from build123d import *

# Parameters (mm, degrees)
SKETCH1_W           = 95
SKETCH1_H           = 83
BOSS_EXTRUDE1_DEPTH = 3
SKETCH3_W           = 95
SKETCH3_H           = 83
SKETCH3_W_2         = 89
SKETCH3_H_2         = 77
BOSS_EXTRUDE2_DEPTH = 9.5
SKETCH4_W           = 6
SKETCH4_H           = 6
BOSS_EXTRUDE3_DEPTH = 9.5
FILLET1_R           = 5
SKETCH5_R           = 1.5
CUT_EXTRUDE1_DEPTH  = 12.5
BOSS_EXTRUDE4_DEPTH = 3
SKETCH7_W           = 12.5
SKETCH7_H           = 3
SKETCH7_W_2         = 10
CUT_EXTRUDE2_DEPTH  = 1.3
SKETCH8_W           = 86
SKETCH8_H           = 5.5
SKETCH8_W_2         = 48.5
SKETCH8_H_2         = 4
SKETCH8_W_3         = 39.36
CUT_EXTRUDE3_DEPTH  = 3
SKETCH10_W          = 10.8
SKETCH10_H          = 3
SKETCH10_W_2        = 13.5
CUT_EXTRUDE4_DEPTH  = 3
SKETCH11_R          = 1.5
CUT_EXTRUDE5_DEPTH  = 3


with BuildPart() as part:
    # Sketch1 → Boss-Extrude1 (new body)
    with BuildSketch(Plane(origin=(0, 0, 0), x_dir=(1, 0, 0), z_dir=(0, 1, 0))):
        with Locations((47.5, 41.5)):
            Rectangle(SKETCH1_W, SKETCH1_H)
    extrude(amount=BOSS_EXTRUDE1_DEPTH)

    # Sketch3 → Boss-Extrude2 (add)
    with BuildSketch(Plane(origin=(0, 3, 0), x_dir=(1, 0, 0), z_dir=(0, 1, 0))):
        with Locations((47.5, 41.5)):
            Rectangle(SKETCH3_W, SKETCH3_H)
        with Locations((47.5, 41.5)):
            Rectangle(SKETCH3_W_2, SKETCH3_H_2, mode=Mode.SUBTRACT)
    extrude(amount=BOSS_EXTRUDE2_DEPTH)

    # Sketch4 → Boss-Extrude3 (add)
    with BuildSketch(Plane(origin=(0, 3, 0), x_dir=(1, 0, 0), z_dir=(0, 1, 0))):
        with Locations((6, 77)):
            Rectangle(SKETCH4_W, SKETCH4_H)
        with Locations((6, 6)):
            Rectangle(SKETCH4_W, SKETCH4_H)
        with Locations((89, 6)):
            Rectangle(SKETCH4_W, SKETCH4_H)
        with Locations((89, 77)):
            Rectangle(SKETCH4_W, SKETCH4_H)
    extrude(amount=BOSS_EXTRUDE3_DEPTH)

    # Fillet1
    fillet1_edges = [part.edges().sort_by_distance(p)[0] for p in [
        (0, 6.25, -83),
        (95, 6.25, -83),
        (95, 6.25, 0),
        (0, 6.25, 0),
    ]]
    fillet(fillet1_edges, radius=FILLET1_R)

    # Sketch5 → Cut-Extrude1 (cut)
    with BuildSketch(Plane(origin=(0, 12.5, 0), x_dir=(1, 0, 0), z_dir=(0, 1, 0))):
        with Locations(Location((5, 78, 0), (0, 0, 270))):
            Circle(SKETCH5_R)
        with Locations(Location((90, 78, 0), (0, 0, 270))):
            Circle(SKETCH5_R)
        with Locations(Location((90, 5, 0), (0, 0, 270))):
            Circle(SKETCH5_R)
        with Locations(Location((5, 5, 0), (0, 0, 270))):
            Circle(SKETCH5_R)
    extrude(amount=-CUT_EXTRUDE1_DEPTH, mode=Mode.SUBTRACT)

    # Sketch6 → Boss-Extrude4 (add)
    with BuildSketch(Plane(origin=(0, 12.5, 0), x_dir=(1, 0, 0), z_dir=(0, 1, 0))):
        with BuildLine():
            Line((5, 0), (90, 0))
            ThreePointArc((90, 0), (93.535533906, 1.464466094), (95, 5))
            Line((95, 5), (95, 78))
            ThreePointArc((95, 78), (93.535533906, 81.535533906), (90, 83))
            Line((90, 83), (5, 83))
            ThreePointArc((5, 83), (1.464466094, 81.535533906), (0, 78))
            Line((0, 78), (0, 5))
            ThreePointArc((0, 5), (1.464466094, 1.464466094), (5, 0))
        make_face()
        with BuildLine():
            Line((5, 1.3), (90, 1.3))
            ThreePointArc((90, 1.3), (92.61629509, 2.38370491), (93.7, 5))
            Line((93.7, 5), (93.7, 78))
            ThreePointArc((93.7, 78), (92.61629509, 80.61629509), (90, 81.7))
            Line((90, 81.7), (5, 81.7))
            ThreePointArc((5, 81.7), (2.38370491, 80.61629509), (1.3, 78))
            Line((1.3, 78), (1.3, 5))
            ThreePointArc((1.3, 5), (2.38370491, 2.38370491), (5, 1.3))
        make_face(mode=Mode.SUBTRACT)
    extrude(amount=BOSS_EXTRUDE4_DEPTH)

    # Sketch7 → Cut-Extrude2 (cut)
    with BuildSketch(Plane.ZY):
        with Locations((-35, 14)):
            Rectangle(SKETCH7_W, SKETCH7_H)
        with Locations((-65.25, 14)):
            Rectangle(SKETCH7_W_2, SKETCH7_H)
    extrude(amount=-CUT_EXTRUDE2_DEPTH, mode=Mode.SUBTRACT)

    # Sketch8 → Cut-Extrude3 (cut)
    with BuildSketch(Plane.XZ):
        with Locations((47.3, -13.65)):
            Rectangle(SKETCH8_W, SKETCH8_H)
        with Locations((44.5, -22.25)):
            Rectangle(SKETCH8_W_2, SKETCH8_H_2)
        with Locations((49.07, -70.5)):
            Rectangle(SKETCH8_W_3, SKETCH8_H_2)
    extrude(amount=-CUT_EXTRUDE3_DEPTH, mode=Mode.SUBTRACT)

    # Sketch10 → Cut-Extrude4 (cut)
    with BuildSketch(Plane.XZ):
        with Locations((15.9, -27.85)):
            Rectangle(SKETCH10_W, SKETCH10_H)
        with Locations((36.05, -27.85)):
            Rectangle(SKETCH10_W_2, SKETCH10_H)
        with Locations((57.35, -27.85)):
            Rectangle(SKETCH10_W_2, SKETCH10_H)
        with Locations((78.65, -27.85)):
            Rectangle(SKETCH10_W_2, SKETCH10_H)
        with Locations((15.9, -50.55)):
            Rectangle(SKETCH10_W, SKETCH10_H)
        with Locations((37.4, -50.55)):
            Rectangle(SKETCH10_W, SKETCH10_H)
        with Locations((57.35, -50.55)):
            Rectangle(SKETCH10_W_2, SKETCH10_H)
        with Locations((78.65, -50.55)):
            Rectangle(SKETCH10_W_2, SKETCH10_H)
    extrude(amount=-CUT_EXTRUDE4_DEPTH, mode=Mode.SUBTRACT)

    # Sketch11 → Cut-Extrude5 (cut)
    with BuildSketch(Plane.XZ):
        with Locations(Location((8, -41.9, 0), (0, 0, 270))):
            Circle(SKETCH11_R)
        with Locations(Location((21.1, -41.9, 0), (0, 0, 270))):
            Circle(SKETCH11_R)
        with Locations(Location((29.5, -41.9, 0), (0, 0, 270))):
            Circle(SKETCH11_R)
        with Locations(Location((42.6, -41.9, 0), (0, 0, 270))):
            Circle(SKETCH11_R)
        with Locations(Location((50.8, -41.9, 0), (0, 0, 270))):
            Circle(SKETCH11_R)
        with Locations(Location((63.9, -41.9, 0), (0, 0, 270))):
            Circle(SKETCH11_R)
        with Locations(Location((72.1, -41.9, 0), (0, 0, 270))):
            Circle(SKETCH11_R)
        with Locations(Location((85.2, -41.9, 0), (0, 0, 270))):
            Circle(SKETCH11_R)
        with Locations(Location((85.2, -64.6, 0), (0, 0, 270))):
            Circle(SKETCH11_R)
        with Locations(Location((72.1, -64.6, 0), (0, 0, 270))):
            Circle(SKETCH11_R)
        with Locations(Location((63.9, -64.6, 0), (0, 0, 270))):
            Circle(SKETCH11_R)
        with Locations(Location((50.8, -64.6, 0), (0, 0, 270))):
            Circle(SKETCH11_R)
        with Locations(Location((42.6, -64.6, 0), (0, 0, 270))):
            Circle(SKETCH11_R)
        with Locations(Location((29.5, -64.6, 0), (0, 0, 270))):
            Circle(SKETCH11_R)
        with Locations(Location((21.1, -64.6, 0), (0, 0, 270))):
            Circle(SKETCH11_R)
        with Locations(Location((8, -64.6, 0), (0, 0, 270))):
            Circle(SKETCH11_R)
    extrude(amount=-CUT_EXTRUDE5_DEPTH, mode=Mode.SUBTRACT)


solid = part.part
The model under review builds one solid part; all positions refer to its coordinate system, in mm. A direction names the side the tool comes from. Round coordinates to 2 decimals unless told otherwise and drop trailing zeros. Loops run counter-clockwise (first coordinate to the right, second up) from the corner with the lowest first, then second, coordinate; pieces in that order, holes last. Notation, with made-up numbers: M 71.25,11 L 99.25,11 A23 ccw 99.25,20 Z; hole C -31.75,33.5 d1. An arc over 180 degrees is marked long. Answer as a JSON object with one key per item and string values.
Item 1: For line 1 along Z through (x, y) = (43.5, 10.5); line 2 along X through (y, z) = (11.75, -25.5); line 3 along Z through (x, y) = (8.5, 3.75), list the stretches that pass through material, from the lowest coordinate up.
Check sheet entries:
{"line 1": "-83 to -80, -3 to 0", "line 2": "0 to 3, 92 to 95", "line 3": "-83 to -74, -9 to 0"}
Item 2: Clearance check with flat-ended pins moving along their axes: P1, Ø12, axis at x = 30, z = -53, coming from the +Y side; P2, Ø2.5, axis at x = 72.1, z = -41.9, coming from the -Y side. State where each tip first meets the part, or that it passes through.
Check sheet entries:
{"P1": "y = 3", "P2": "through"}
Item 3: We need section C-C, the plane z = -17.5. State the section outline as (x, y) points, and give its area (3 significant figures).
Check sheet entries:
{"outline": "M 0,0 L 95,0 L 95,15.5 L 93.7,15.5 L 93.7,12.5 L 92,12.5 L 92,3 L 3,3 L 3,12.5 L 1.3,12.5 L 1.3,15.5 L 0,15.5 Z", "area": "350 mm2"}
Item 4: We need section B-B, the plane y = 10.75. State the section outline as (x, z) points.
Check sheet entries:
{"outline": "M 0,-78 A5 ccw 5,-83 L 90,-83 A5 ccw 95,-78 L 95,-5 A5 ccw 90,0 L 5,0 A5 ccw 0,-5 Z; hole M 3,-74 L 9,-74 L 9,-80 L 86,-80 L 86,-74 L 92,-74 L 92,-9 L 86,-9 L 86,-3 L 9,-3 L 9,-9 L 3,-9 Z; hole C 5,-78 d3; hole C 5,-5 d3; hole C 90,-78 d3; hole C 90,-5 d3"}
Item 5: Tool access review of faces 3 (the face through (21.3, 1, -28)), 4 (the face through (3, 8, -41)): name each direction out of +Z, -Z, +X, -X, +Y, -Y from which nothing blocks a thin tool from reaching the whole face with its end or side.
Check sheet entries:
{"face 3": "+Y, -Y", "face 4": "+Y"}
Item 6: We need section D-D, the plane z = -64.6. State how many separate pieces and enclosed holes the cut face has, and give its area (3 significant figures).
Check sheet entries:
{"separate pieces": "9", "enclosed holes": "0", "area": "274 mm2"}
Item 7: We need section A-A, the plane x = 82.5. State the section outline as (y, z) points.
Check sheet entries:
{"outline": "M 0,-83 L 15.5,-83 L 15.5,-81.7 L 12.5,-81.7 L 12.5,-80 L 3,-80 L 3,-52.05 L 0,-52.05 Z; M 0,-49.05 L 3,-49.05 L 3,-29.35 L 0,-29.35 Z; M 0,-26.35 L 3,-26.35 L 3,-16.4 L 0,-16.4 Z; M 0,-10.9 L 3,-10.9 L 3,-3 L 12.5,-3 L 12.5,-1.3 L 15.5,-1.3 L 15.5,0 L 0,0 Z"}
Item 8: The part is to be moulded in two halves that separate along X. For faces 1 (the face through (91.265, 6.338, -77.194)), 2 (the face through (47, 0, -42)), say which applies: +X half, -X half, draft (parallel to the pull), parting line (faces both ways), or undercut.
Check sheet entries:
{"face 1": "undercut", "face 2": "draft"}
